```python
from build123d import *

# Parameters (mm, degrees)
SKETCH_2_R           = 3.05
SKETCH_2_R_2         = 1.55
EXTRUDE_1_DEPTH      = 25
CUT_EXTRUDE_3_DEPTH  = 74.430746455
SKETCH_8_R           = 1.6
CUT_EXTRUDE_4_DEPTH  = 0.8
CUT_EXTRUDE_START    = -2.895
CUT_EXTRUDE_10_DEPTH = 6.1


# Read off the part's stored shape, not the designer's step: the extrude step
with BuildPart() as part:
    # 草图2 → 凸台-拉伸1 (new body)
    # profile 1 of 4: a face of its own
    with BuildSketch(Plane.XY.offset(70)):
        with Locations((-18.9, 15.755)):
            Circle(SKETCH_2_R)
        with Locations((-18.9, 15.755)):
            Circle(SKETCH_2_R_2, mode=Mode.SUBTRACT)
    # profile 2 of 4: a face of its own
    with BuildSketch(Plane.XY.offset(70)):
        with BuildLine():
            Line((0, 12.705), (0, 15.6))
            Line((0, 15.6), (-15.853941071, 15.6))
            ThreePointArc((-15.853941071, 15.6), (-16.798839606, 13.544202633), (-18.9, 12.705))
            Line((-18.9, 12.705), (0, 12.705))
        make_face()
    # profile 3 of 4: a face of its own
    with BuildSketch(Plane.XY.offset(70)):
        with BuildLine():
            Line((15.853941071, 15.6), (0, 15.6))
            Line((0, 15.6), (0, 12.705))
            Line((0, 12.705), (18.9, 12.705))
            ThreePointArc((18.9, 12.705), (16.798839606, 13.544202633), (15.853941071, 15.6))
        make_face()
    # profile 4 of 4: a face of its own
    with BuildSketch(Plane.XY.offset(70)):
        with Locations((18.9, 15.755)):
            Circle(SKETCH_2_R)
        with Locations((18.9, 15.755)):
            Circle(SKETCH_2_R_2, mode=Mode.SUBTRACT)
    extrude(amount=-EXTRUDE_1_DEPTH)

    # 草图7 → 切除-拉伸3 (cut, through all)
    with BuildSketch(Plane(origin=(0, 15.6, 0), x_dir=(1, 0, 0), z_dir=(0, 1, 0))):
        with BuildLine():
            Line((0.25, -50.75), (-0.25, -50.75))
            ThreePointArc((-0.25, -50.75), (-1, -50), (-0.25, -49.25))
            Line((-0.25, -49.25), (0.25, -49.25))
            ThreePointArc((0.25, -49.25), (1, -50), (0.25, -50.75))
        make_face()
    extrude(amount=-CUT_EXTRUDE_3_DEPTH, mode=Mode.SUBTRACT)

    # 草图8 → 切除-拉伸4 (cut)
    with BuildSketch(Plane.XZ.offset(-12.705)):
        with Locations((0, 50)):
            Circle(SKETCH_8_R)
    extrude(amount=-CUT_EXTRUDE_4_DEPTH, mode=Mode.SUBTRACT)

    # 切除-拉伸10 outline → 切除-拉伸10 (cut)
    with BuildSketch(Plane(origin=(0, 15.6, 0), x_dir=(1, 0, 0), z_dir=(0, 1, 0)).offset(CUT_EXTRUDE_START)):
        Polygon((-6.666660498, -57), (-21.95, -57), (-21.95, -70), (15.85, -70), align=None)
        Polygon((-21.95, -50), (-10.853941071, -50), (-2.193687033, -45), (-21.95, -45), align=None)
        Polygon((10.853941071, -50), (21.95, -50), (21.95, -45), (2.193687033, -45), align=None)
    extrude(amount=CUT_EXTRUDE_10_DEPTH, mode=Mode.SUBTRACT)


solid = part.part
```
Check sheet for the modelled part. Datum: model origin and axes. Units: mm. A direction names the side the tool comes from. Round coordinates to 2 decimals unless told otherwise and drop trailing zeros. Order: outer loops, then holes, each group sorted by start corner. A loop starts at its lowest first (then second) coordinate and runs counter-clockwise, first axis right, second up.
1) Tool access check on faces 1 (the cylindrical face through (1, 15, 50)), 2 (the flat face through (-14, 15, 57)), 3 (the flat face through (16, 15, 50)). Record the directions out of +Z, -Z, +X, -X, +Y, -Y that give a thin tool (end or side, any length) a straight path to the whole face; none if there is none.
2) Section check A-A (y = 18). Record the boundary of the cut face in (x, z).
3) Section check B-B (z = 68.25). Record the boundary of the cut face in (x, y) (3 decimals).
4) Mould release check, pull along X, two halves, no side actions. Record for faces 4 (the flat face through (-6.584, 14.132, 47.535)), 5 (the cylindrical face through (0.86, 13.1, 51.35)), 6 (the flat face through (4, 15.6, 55)), 7 (the flat face through (18, 14, 70)): +X half, -X half, draft (parallel to the pull), parting line (faces both ways), or undercut.
5) Scan lines: line 1 (Y direction, x = -18.9, z = 53.5) (3 decimals); line 2 (X direction, y = 15.75, z = 61.75); line 3 (X direction, y = 15, z = 53.75). Record each from-to range of solid material in increasing order.
6) Section check C-C (x = 7). Record the boundary of the cut face in (y, z) (3 decimals), and give its area (3 significant figures).
7) Go/stop test with flat-tipped pins: pin 1 Ø3 at (x, z) = (16.5, 67) entering from +Y; pin 2 Ø1.6 at (x, z) = (0.5, 50) entering from -Y (3 decimals); pin 3 Ø2 at (x, z) = (5.5, 64.5) entering from +Y. Record where each tip stops, or that it passes through.
Result:
1. face 1: +Y, -Y
1. face 2: +Z, -X, +Y, -Y
1. face 3: -Z, +X, +Y, -Y
2. outline: (-20.96, 50) - (-16.84, 50) - (-16.84, 57) - (-20.96, 57) - close; (16.84, 50) - (20.96, 50) - (20.96, 70) - (16.84, 70) - close
3. outline: (12.819, 12.705) - (18.9, 12.705) arc R3.05 ccw (long way) to (15.854, 15.6) - (12.819, 15.6) - close; hole circle Ø3.1 at (18.9, 15.755)
4. face 4: -X half
4. face 5: undercut
4. face 6: undercut
4. face 7: draft
5. line 1: y = 12.705 to 14.205, 17.305 to 18.805
5. line 2: x = 15.85 to 17.35, 20.45 to 21.95
5. line 3: x = -21.86 to -20.25, -17.55 to 17.55, 20.25 to 21.86
6. outline: (12.705, 47.775) - (15.6, 47.775) - (15.6, 64.89) - (12.705, 64.89) - close
6. area: 49.5 mm2
7. pin 1: stops at y = 18.67
7. pin 2: stops at y = 13.505
7. pin 3: stops at y = 15.6
